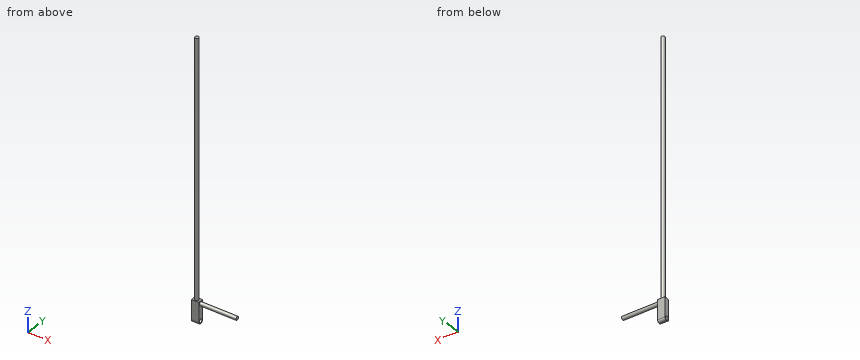
from build123d import *

# Parameters (mm, degrees)
SKETCH1_W           = 10
SKETCH1_H           = 7
BOSS_EXTRUDE1_DEPTH = 30
SKETCH2_R           = 2.5
CUT_EXTRUDE2_DEPTH  = 20
SKETCH2_3_R         = 2.5
BOSS_EXTRUDE2_DEPTH = 50
FILLET1_R           = 3
SKETCH3_R           = 2.5
BOSS_EXTRUDE3_DEPTH = 350


with BuildPart() as part:
    # Sketch1 → Boss-Extrude1 (new body)
    with BuildSketch(Plane.XY):
        Rectangle(SKETCH1_W, SKETCH1_H)
    extrude(amount=BOSS_EXTRUDE1_DEPTH)

    # Sketch2 → Cut-Extrude2 (cut)
    with BuildSketch(Plane(origin=(5, 0, 0), x_dir=(0, 0, -1), z_dir=(1, 0, 0))):
        with Locations(Location((-3.5, 0, 0), (0, 0, 90))):
            Circle(SKETCH2_R)
    extrude(amount=-CUT_EXTRUDE2_DEPTH, mode=Mode.SUBTRACT)

    # Sketch2_3 → Boss-Extrude2 (add)
    with BuildSketch(Plane(origin=(5, 0, 0), x_dir=(0, 0, -1), z_dir=(1, 0, 0))):
        with Locations(Location((-26.5, 0, 0), (0, 0, 180))):
            Circle(SKETCH2_3_R)
    extrude(amount=BOSS_EXTRUDE2_DEPTH)

    # Fillet1
    fillet1_edges = [part.edges().sort_by_distance(p)[0] for p in [
        (0, -3.5, 0),
        (0, 3.5, 0),
    ]]
    fillet(fillet1_edges, radius=FILLET1_R)

    # Sketch3 → Boss-Extrude3 (add)
    with BuildSketch(Plane.XY.offset(30)):
        Circle(SKETCH3_R)
    extrude(amount=BOSS_EXTRUDE3_DEPTH)


solid = part.part
Input: part model. Units: mm. Frame: model coordinates. Round coordinates to 2 decimals unless told otherwise and drop trailing zeros. Write each loop counter-clockwise with the first axis right and the second up, starting at its lowest first coordinate (ties: lowest second). Pieces come first, ordered by that corner, then holes.
1) Cut plane B-B (z = 257). Return the cut outline in (x, y).
2) Cut plane A-A (x = 33). Return the cut outline in (y, z), then the cut area to 3 significant figures.
3) Ray query, L1, parallel to Y at x = -2, z = 3; L2, parallel to Z at x = -2.25, y = 0; L3, parallel to X at y = -2.5, z = 20.5. Return the intervals inside material, ascending.
4) Contact query for flat-ended pins moving along their axis: P1, Ø4, axis at x = 12.5, y = -1, coming from the -Z side; P2, Ø2, axis at y = -2, z = 67.5, coming from the -X side. Output: stop coordinate, or through.
Geometry says:
1. outline: circle Ø5 at (0, 0)
2. outline: circle Ø5 at (0, 26.5)
2. area: 19.6 mm2
3. L1: y = -3.5 to -2.45, 2.45 to 3.5
3. L2: z = 0 to 1, 6 to 380
3. L3: x = -5 to 5
4. P1: stops at z = 24
4. P2: stops at x = -2.29
